```python
from build123d import *

# Parameters (mm, degrees)
F0_R     = 35
F2_R     = 75
F4_R     = 35
F5_DEPTH = 18
F7_T     = -2.5


# Not quite as in the source:
# - a fillet or chamfer that OpenCascade refuses, or shapes differently, is made with other operations: its cross-section is extruded or revolved along the edge and cut away or added


with BuildPart() as f3:
    # F0 (on Top) → F3 section 0
    with BuildSketch(Plane.XY):
        Circle(F0_R)
    # F2 (on offset) → F3 section 1
    with BuildSketch(Plane.XY.offset(21)):
        Circle(F2_R)
    loft()

    # F4 (on face) → F5 (cut)
    with BuildSketch(Plane(origin=(0, 0, 0), x_dir=(1, 0, 0), z_dir=(0, 0, -1))):
        Circle(F4_R)
    extrude(amount=-F5_DEPTH, mode=Mode.SUBTRACT)

    # F6: chamfer of 18 on 1 edges, made by hand


with BuildPart() as f6_tool2:
    # F6_s3 → F6_t4 (revolve)
    with BuildSketch(Plane.XZ):
        Polygon((50.9371622511, 8.3670101818), (35, 18), (35, 0), align=None)
    revolve(axis=Axis((0, 0, 0), (0, 0, 1)))

    split(bisect_by=Plane.XY.offset(18), keep=Keep.BOTTOM)


with BuildPart() as f3_1:
    add(f3.part)

    # F6_t1: cut F6_tool2
    add(f6_tool2.part, mode=Mode.SUBTRACT)

    # F7
    f7_openings = [f3_1.faces().sort_by_distance(p)[0] for p in [
        (0, 0, 21),
    ]]
    offset(amount=F7_T, openings=f7_openings, kind=Kind.INTERSECTION)


solid = f3_1.part
```
Verification items for the finished model (mm, model axes). A direction names the side the tool comes from. Give positions to 0.01 mm unless a question says otherwise; leave off trailing zeros. Order: outer loops, then holes, each group sorted by start corner. A loop starts at its lowest first (then second) coordinate and runs counter-clockwise, first axis right, second up. Notation, with made-up numbers: (68, 53) -> (109, 53) arc R35 cw to (109, 85) -> close; hole circle Ø5 at (36.25, -20). An arc over 180 degrees is marked (long way). Use a Markdown table: item, result.
1) Section check B-B, the plane z = 15.5. Record the boundary of the cut face in (x, y).
Results:
| item | result |
|---|---|
| outline | circle Ø129.05 at (0, 0); circle Ø87.94 at (0, 0); hole circle Ø118.29 at (0, 0); hole circle Ø78.27 at (0, 0) |
2) Section check A-A, the plane x = 0. Record the boundary of the cut face in (y, z).
Results:
| item | result |
|---|---|
| outline | (-75, 21) -> (-50.94, 8.37) -> (-35, 18) -> (35, 18) -> (50.94, 8.37) -> (75, 21) -> (69.62, 21) -> (51.02, 11.24) -> (35.7, 20.5) -> (-35.7, 20.5) -> (-51.02, 11.24) -> (-69.62, 21) -> close |
3) Depth check by flat-ended pin: pin 1 Ø4 at (x, z) = (17.5, 10) entering from +Y; pin 2 Ø12 at (x, y) = (-19, -37) entering from +Z; pin 3 Ø21 at (x, y) = (0, -8.5) entering from -Z. Enter the tip coordinate at first touch or a pass-through.
Results:
| item | result |
|---|---|
| pin 1 | y = 55.2 |
| pin 2 | z = 20.5 |
| pin 3 | z = 18 |
4) Mould release check, pull along X, two halves, no side actions. Record for faces 1 (the conical face through (34.76, 10.95, 20.05)), 2 (the conical face through (-11.37, -51.2, 9.16)), 3 (the flat face through (21.9, -66.3, 21)): pulls with the +X half, pulls with the -X half, needs draft (parallel to the pull), parting line crosses it, or undercut.
Results:
| item | result |
|---|---|
| face 1 | undercut |
| face 2 | parting line crosses it |
| face 3 | needs draft |
5) Tool access check on faces 4 (the flat face through (0, 0, 20.5)), 5 (the flat face through (0, 0, 18)). Record the directions out of +Z, -Z, +X, -X, +Y, -Y that give a thin tool (end or side, any length) a straight path to the whole face; none if there is none.
Results:
| item | result |
|---|---|
| face 4 | +Z |
| face 5 | -Z |
6) Material ranges on probe 1 along Y at (x, z) = (23, 19.25); probe 2 along Y at (x, z) = (-10.5, 11.75); probe 3 along X at (y, z) = (-20, 19.5), recorded low to high.
Results:
| item | result |
|---|---|
| probe 1 | -67.88 to -62.17, -29.95 to 29.95, 62.17 to 67.88 |
| probe 2 | -56.41 to -50.93, -49.06 to -44.11, 44.11 to 49.06, 50.93 to 56.41 |
| probe 3 | -69.32 to -63.7, -31.55 to 31.55, 63.7 to 69.32 |
